```python
from build123d import *

# Parameters (mm, degrees)
SKETCH211_R   = 3.25
PAD055_DEPTH  = 5
SKETCH212_W   = 4
SKETCH212_H   = 6
SKETCH212_W_2 = 6
SKETCH212_H_2 = 4
PAD056_DEPTH  = 5
CHAMFER_SIZE  = 0.45


with BuildPart() as endstopper:
    # Sketch211 → Pad055 (new body)
    with BuildSketch(Plane.XZ):
        with BuildLine():
            Line((9, 10), (-19, 10))
            ThreePointArc((-19, 10), (-19.707107, 9.707107), (-20, 9))
            Line((-20, 9), (-20, -24))
            ThreePointArc((-20, -24), (-19.707107, -24.707107), (-19, -25))
            Line((-19, -25), (-11, -25))
            ThreePointArc((-11, -25), (-10.292893, -24.707107), (-10, -24))
            Line((-10, -24), (-10, -15))
            ThreePointArc((-5, -10), (-8.535534, -11.464466), (-10, -15))
            Line((-5, -10), (9, -10))
            ThreePointArc((9, -10), (9.707107, -9.707107), (10, -9))
            Line((10, 9), (10, -9))
            ThreePointArc((10, 9), (9.707107, 9.707107), (9, 10))
        make_face()
        Circle(SKETCH211_R, mode=Mode.SUBTRACT)
    extrude(amount=-PAD055_DEPTH)

    # Sketch212 → Pad056 (join)
    with BuildSketch(Plane.XZ):
        with Locations((-8, 0)):
            Rectangle(SKETCH212_W, SKETCH212_H)
        with Locations((8, 0)):
            Rectangle(SKETCH212_W, SKETCH212_H)
        with Locations((0, -8)):
            Rectangle(SKETCH212_W_2, SKETCH212_H_2)
    extrude(amount=PAD056_DEPTH)

    # Chamfer
    chamfer_edges = [endstopper.edges().sort_by_distance(p)[0] for p in [
        (9.707107, 5, 9.707107),
        (-5, 5, 10),
        (-19.707107, 5, 9.707107),
        (-20, 5, -7.5),
        (-19.707107, 5, -24.707107),
        (-15, 5, -25),
        (-10.292893, 5, -24.707107),
        (-10, 5, -19.5),
        (-8.535534, 5, -11.464466),
        (2, 5, -10),
        (9.707107, 5, -9.707107),
        (10, 5, 0),
        (-3.25, 5, 0),
    ]]
    chamfer(chamfer_edges, length=CHAMFER_SIZE)


with BuildPart() as endstopper_1:
    # Body022046 placement: moved
    add(endstopper.part.moved(Location((-113, 123, -62))))


with BuildPart() as endstopper_m:
    # Part__Mirroring: instance of EndStopper
    add(endstopper_1.part.mirror(Plane(origin=(0, 0, 0), x_dir=(0, -1, 0), z_dir=(1, 0, 0))))


solid = endstopper_m.part
```
Here's how the part is built. I have some questions about the finished solid (model axes, mm). A direction names the side the tool comes from. Give positions to 0.01 mm unless a question says otherwise; leave off trailing zeros. Loops run counter-clockwise (first coordinate to the right, second up) from the corner with the lowest first, then second, coordinate; pieces in that order, holes last. Notation, with made-up numbers: M 67.5,-27 L 122.5,-27 A18 cw 122.5,-21 Z; hole C -40,-38 d10. An arc over 180 degrees is marked long. Put each result on its own line as item: value. Start each with the question number.
(1) Will these pins go through, and if not, where does the flat tip stop? pin 1 Ø5.5 at (y, z) = (119.5, -61.5) entering from +X; pin 2 Ø5 at (x, y) = (110, 121) entering from -Z; pin 3 Ø2.5 at (x, y) = (114, 120) entering from +Z.
(2) I want a section at D-D on y = 119.5. Please give me the cut outline in (x, z), then the cut area to 3 significant figures.
(3) For faces 1 (the flat face through (110, 121, -70)), 2 (the flat face through (121, 121, -59)), 3 (the flat face through (123, 125, -82)), which set-ups out of +Z, -Z, +X, -X, +Y, -Y let a thin tool reach every point of the face, with its end or its side?
(4) I want a section at A-A on y = 127. Please give me the cut outline in (x, z), then the cut area to 3 significant figures.
(5) I want a section at C-C on z = -62. Please give me the cut outline in (x, y).
(6) I want a section at B-B on x = 113. Please give me the cut outline in (y, z), then the cut area to 3 significant figures.
(7) I need wall thicknesses on line 1 along X through (y, z) = (120.25, -62.5); line 2 along Z through (x, y) = (113, 124.55); line 3 along Y through (x, z) = (125, -71). Which ranges of each line are inside material? Lowest first, please. Write a range as [from, to].
Answer block:
1. pin 1: x = 123
1. pin 2: z = -72
1. pin 3: z = -68
2. outline: M 103,-65 L 107,-65 L 107,-59 L 103,-59 Z; M 110,-72 L 116,-72 L 116,-68 L 110,-68 Z; M 119,-65 L 123,-65 L 123,-59 L 119,-59 Z
2. area: 72.0 mm^2
3. face 1: +Z, -Z, -X, -Y
3. face 2: +Z, +X, -X, -Y
3. face 3: -Z, -X, +Y, -Y
4. outline: M 103,-71 A1 ccw 104,-72 L 118,-72 A5 cw 123,-77 L 123,-86 A1 ccw 124,-87 L 132,-87 A1 ccw 133,-86 L 133,-53 A1 ccw 132,-52 L 104,-52 A1 ccw 103,-53 Z; hole C 113,-62 d6.5
4. area: 721 mm^2
5. outline: M 103,118 L 107,118 L 107,123 L 109.75,123 L 109.75,127.55 L 109.3,128 L 103.45,128 L 103,127.55 Z; M 116.25,123 L 119,123 L 119,118 L 123,118 L 123,123 L 133,123 L 133,127.55 L 132.55,128 L 116.7,128 L 116.25,127.55 Z
6. outline: M 118,-72 L 127.55,-72 L 128,-71.55 L 128,-65.7 L 127.55,-65.25 L 123,-65.25 L 123,-68 L 118,-68 Z; M 123,-58.75 L 127.55,-58.75 L 128,-58.3 L 128,-52.45 L 127.55,-52 L 123,-52 Z
6. area: 87.1 mm^2
7. line 1: [103, 107], [119, 123]
7. line 2: [-72, -65.25], [-58.75, -52]
7. line 3: [123, 128]
